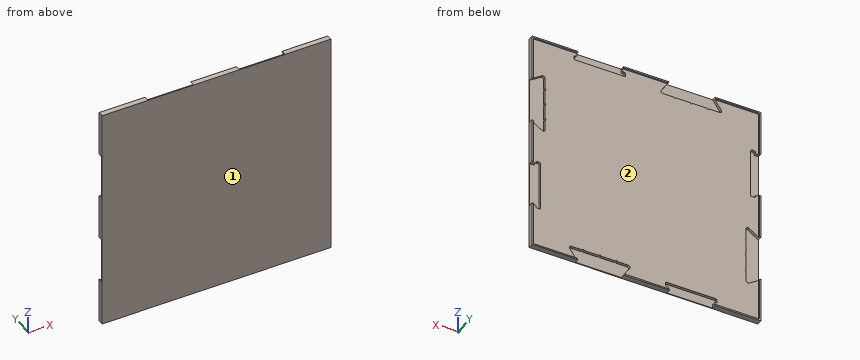
```python
from build123d import *

# Parameters (mm, degrees)
SKETCH1_W           = 250
SKETCH1_H           = 250
BOSS_EXTRUDE1_DEPTH = 2.875
SKETCH2_W           = 247
SKETCH2_H           = 247
CUT_EXTRUDE1_DEPTH  = 1.75
CUT_EXTRUDE2_START  = -4.75
CUT_EXTRUDE2_DEPTH  = 182.620185447
CUT_EXTRUDE4_DEPTH  = 3
CUT_EXTRUDE3_START  = -4.75
CUT_EXTRUDE3_DEPTH  = 182.620185447
FILLET2_R           = 1
FILLET3_R           = 2
CIRPATTERN1_START   = -1.875
CIRPATTERN1_DEPTH   = 4.75


# Read off the part's stored shape, not the designer's step: CirPattern1
with BuildPart() as part:
    # Sketch1 → Boss-Extrude1 (new, symmetric)
    with BuildSketch(Plane(origin=(0, 0, 0), x_dir=(1, 0, 0), z_dir=(0, 1, 0))):
        Rectangle(SKETCH1_W, SKETCH1_H)
    extrude(amount=BOSS_EXTRUDE1_DEPTH, both=True)

    # Sketch2 → Cut-Extrude1 (cut)
    with BuildSketch(Plane(origin=(0, 2.875, 0), x_dir=(1, 0, 0), z_dir=(0, 1, 0))):
        Rectangle(SKETCH2_W, SKETCH2_H)
    extrude(amount=-CUT_EXTRUDE1_DEPTH, mode=Mode.SUBTRACT)

    # Sketch4 → Cut-Extrude2 (cut)
    with BuildSketch(Plane(origin=(0, 2.875, 0), x_dir=(1, 0, 0), z_dir=(0, 1, 0)).offset(CUT_EXTRUDE2_START)):
        Polygon((-75, -125), (-85, -110), (-15, -110), (-25, -125), align=None)
    extrude(amount=CUT_EXTRUDE2_DEPTH, mode=Mode.SUBTRACT)

    # Sketch6 → Cut-Extrude4 (cut)
    with BuildSketch(Plane(origin=(0, 1.125, 0), x_dir=(1, 0, 0), z_dir=(0, 1, 0))):
        with BuildLine():
            Line((-69, -110), (-67, -110))
            ThreePointArc((-67, -110), (-68, -109), (-69, -110))
        make_face()
        with BuildLine():
            Line((-51, -110), (-49, -110))
            ThreePointArc((-49, -110), (-50, -109), (-51, -110))
        make_face()
        with BuildLine():
            Line((-33, -110), (-31, -110))
            ThreePointArc((-31, -110), (-32, -109), (-33, -110))
        make_face()
    extrude(amount=-CUT_EXTRUDE4_DEPTH, mode=Mode.SUBTRACT)

    # Sketch5 → Cut-Extrude3 (cut)
    with BuildSketch(Plane(origin=(0, 2.875, 0), x_dir=(1, 0, 0), z_dir=(0, 1, 0)).offset(CUT_EXTRUDE3_START)):
        Polygon((25, -125), (25, -120), (22, -120), (22, -115), (78, -115), (78, -120), (75, -120), (75, -125), align=None)
    extrude(amount=CUT_EXTRUDE3_DEPTH, mode=Mode.SUBTRACT)

    # Fillet2
    fillet2_edges = [part.edges().sort_by_distance(p)[0] for p in [
        (-123.5, 2, -123.5),
        (-123.5, 2, 123.5),
        (123.5, 2, 123.5),
        (123.5, 2, -123.5),
        (75, -0.375, 120),
        (78, -0.375, 120),
        (78, -0.375, 115),
        (22, -0.375, 115),
        (22, -0.375, 120),
        (25, -0.375, 120),
    ]]
    fillet(fillet2_edges, radius=FILLET2_R)

    # Fillet3
    fillet3_edges = [part.edges().sort_by_distance(p)[0] for p in [
        (-85, -0.375, 110),
        (-15, -0.375, 110),
    ]]
    fillet(fillet3_edges, radius=FILLET3_R)

    # CirPattern1 outline → CirPattern1 (cut)
    with BuildSketch(Plane(origin=(0, 0, 0), x_dir=(1, 0, 0), z_dir=(0, 1, 0)).offset(CIRPATTERN1_START)):
        with BuildLine():
            ThreePointArc((110, -31), (109, -32), (110, -33))
            Line((110, -33), (110, -49))
            ThreePointArc((110, -49), (109, -50), (110, -51))
            Line((110, -51), (110, -67))
            ThreePointArc((110, -67), (109, -68), (110, -69))
            Line((110, -69), (110, -81.262965816))
            ThreePointArc((110, -81.262965816), (111.056284149, -83.026315014), (113.109400392, -82.927066405))
            Line((113.109400392, -82.927066405), (125, -75))
            Line((125, -75), (125, -25))
            Line((125, -25), (113.109400392, -17.072933595))
            ThreePointArc((113.109400392, -17.072933595), (111.056284149, -16.973684986), (110, -18.737034184))
            Line((110, -18.737034184), (110, -31))
        make_face()
        with BuildLine():
            Line((-125, 75), (-125, 25))
            Line((-125, 25), (-113.109400392, 17.072933595))
            ThreePointArc((-113.109400392, 17.072933595), (-111.056284149, 16.973684986), (-110, 18.737034184))
            Line((-110, 18.737034184), (-110, 31))
            ThreePointArc((-110, 31), (-109, 32), (-110, 33))
            Line((-110, 33), (-110, 49))
            ThreePointArc((-110, 49), (-109, 50), (-110, 51))
            Line((-110, 51), (-110, 67))
            ThreePointArc((-110, 67), (-109, 68), (-110, 69))
            Line((-110, 69), (-110, 81.262965816))
            ThreePointArc((-110, 81.262965816), (-111.056284149, 83.026315014), (-113.109400392, 82.927066405))
            Line((-113.109400392, 82.927066405), (-125, 75))
        make_face()
        with BuildLine():
            Line((75, 125), (25, 125))
            Line((25, 125), (17.072933595, 113.109400392))
            ThreePointArc((17.072933595, 113.109400392), (16.973684986, 111.056284149), (18.737034184, 110))
            Line((18.737034184, 110), (31, 110))
            ThreePointArc((31, 110), (32, 109), (33, 110))
            Line((33, 110), (49, 110))
            ThreePointArc((49, 110), (50, 109), (51, 110))
            Line((51, 110), (67, 110))
            ThreePointArc((67, 110), (68, 109), (69, 110))
            Line((69, 110), (81.262965816, 110))
            ThreePointArc((81.262965816, 110), (83.026315014, 111.056284149), (82.927066405, 113.109400392))
            Line((82.927066405, 113.109400392), (75, 125))
        make_face()
        with BuildLine():
            Line((125, 75), (121, 75))
            ThreePointArc((121, 75), (120.292893219, 75.292893219), (120, 76))
            Line((120, 76), (120, 77))
            ThreePointArc((120, 77), (119.707106781, 77.707106781), (119, 78))
            Line((119, 78), (116, 78))
            ThreePointArc((116, 78), (115.292893219, 77.707106781), (115, 77))
            Line((115, 77), (115, 23))
            ThreePointArc((115, 23), (115.292893219, 22.292893219), (116, 22))
            Line((116, 22), (119, 22))
            ThreePointArc((119, 22), (119.707106781, 22.292893219), (120, 23))
            Line((120, 23), (120, 24))
            ThreePointArc((120, 24), (120.292893219, 24.707106781), (121, 25))
            Line((121, 25), (125, 25))
            Line((125, 25), (125, 75))
        make_face()
        with BuildLine():
            Line((-25, 125), (-75, 125))
            Line((-75, 125), (-75, 121))
            ThreePointArc((-75, 121), (-75.292893219, 120.292893219), (-76, 120))
            Line((-76, 120), (-77, 120))
            ThreePointArc((-77, 120), (-77.707106781, 119.707106781), (-78, 119))
            Line((-78, 119), (-78, 116))
            ThreePointArc((-78, 116), (-77.707106781, 115.292893219), (-77, 115))
            Line((-77, 115), (-23, 115))
            ThreePointArc((-23, 115), (-22.292893219, 115.292893219), (-22, 116))
            Line((-22, 116), (-22, 119))
            ThreePointArc((-22, 119), (-22.292893219, 119.707106781), (-23, 120))
            Line((-23, 120), (-24, 120))
            ThreePointArc((-24, 120), (-24.707106781, 120.292893219), (-25, 121))
            Line((-25, 121), (-25, 125))
        make_face()
        with BuildLine():
            Line((-125, -25), (-125, -75))
            Line((-125, -75), (-121, -75))
            ThreePointArc((-121, -75), (-120.292893219, -75.292893219), (-120, -76))
            Line((-120, -76), (-120, -77))
            ThreePointArc((-120, -77), (-119.707106781, -77.707106781), (-119, -78))
            Line((-119, -78), (-116, -78))
            ThreePointArc((-116, -78), (-115.292893219, -77.707106781), (-115, -77))
            Line((-115, -77), (-115, -23))
            ThreePointArc((-115, -23), (-115.292893219, -22.292893219), (-116, -22))
            Line((-116, -22), (-119, -22))
            ThreePointArc((-119, -22), (-119.707106781, -22.292893219), (-120, -23))
            Line((-120, -23), (-120, -24))
            ThreePointArc((-120, -24), (-120.292893219, -24.707106781), (-121, -25))
            Line((-121, -25), (-125, -25))
        make_face()
    extrude(amount=CIRPATTERN1_DEPTH, mode=Mode.SUBTRACT)


solid = part.part
```
The model under review builds one solid part; all positions refer to its coordinate system, in mm. Face numbers are marked on the shaded views. Round coordinates to 2 decimals unless told otherwise and drop trailing zeros. Loops run counter-clockwise (first coordinate to the right, second up) from the corner with the lowest first, then second, coordinate; pieces in that order, holes last.
1) Wall thickness on line 1 along Z through (x, y) = (-10, 1.45); line 2 along Y through (x, z) = (74.5, -77) (3 decimals): over which ranges is each line inside the solid? List them lowest first.
Values follow:
line 1: z = -125 to -123.5, 123.5 to 125
line 2: y = -2.875 to 1.125
2) Consider section A-A on z = -36. State the section outline as (x, y) points (3 decimals), then the cut area to 3 significant figures.
Values follow:
outline: (-125, -2.875) - (125, -2.875) - (125, -1.875) - (115, -1.875) - (115, 1.125) - (-110, 1.125) - (-110, -1.875) - (-125, -1.875) - close
area: 925 mm2
3) Consider section B-B on x = -104. State the section outline as (y, z) points (3 decimals), then the cut area to 3 significant figures.
Values follow:
outline: (-2.875, -125) - (2.875, -125) - (2.875, -123.5) - (1.125, -123.5) - (1.125, 123.5) - (2.875, 123.5) - (2.875, 125) - (-2.875, 125) - close
area: 1,010 mm2
4) Clearance check with flat-ended pins moving along their axes: P1, Ø6, axis at x = -83, z = -84, coming from the +Y side (3 decimals); P2, Ø2.5, axis at y = -0.5, z = -72.5, coming from the -X side; P3, Ø2.5, axis at x = 61.5, y = -0.5, coming from the -Z side. State where each tip first meets the part, or that it passes through.
Values follow:
P1: stops at y = 1.125
P2: stops at x = -110
P3: stops at z = -110
5) The part is to be moulded in two halves that separate along X. For the marked faces 1 and 2, say which applies: pulls with the +X half, pulls with the -X half, needs draft (parallel to the pull), parting line crosses it, or undercut.
Values follow:
face 1: needs draft
face 2: undercut
